Geometry: final body of the model. Coordinates: model frame, mm. A direction names the side the tool comes from. Give positions to 0.01 mm unless a question says otherwise; leave off trailing zeros. Loops run counter-clockwise (first coordinate to the right, second up) from the corner with the lowest first, then second, coordinate; pieces in that order, holes last. Notation, with made-up numbers: (44, 24.5) -> (77, 24.5) arc R24 ccw to (77, 56.5) -> close; hole circle Ø3 at (1, 30). An arc over 180 degrees is marked (long way). Answer in a Markdown table with one row per item. Add a question column.
1) Line query: line 1 (X direction, y = 110, z = 2.9); line 2 (Y direction, x = -268, z = 5.45); line 3 (Y direction, x = -479, z = 2.7). Output: solid intervals per line, ascending. Write a range as from..to.
2) Section query D-D (y = 147). Return the cut outline in (x, z).
3) Section query B-B (x = -372). Return the cut outline in (y, z).
4) First-contact query: P1, Ø2, axis at y = 257, z = 2, coming from the -X side; P2, Ø1.8, axis at y = 100.5, z = 4, coming from the +X side; P3, Ø2, axis at y = 307.5, z = 1, coming from the +X side. Flat tips, straight axial feed; report the tip coordinate or a pass-through.
5) Access query for faces 1 (the flat face through (-345, 205, 6)), 2 (the flat face through (-416.64, 252.094, 2.958)). Directions: +Z, -Z, +X, -X, +Y, -Y. A direction counts if a zero-diameter tool reaches every point of the face in a straight line with its end or side. Return the directions, or none.
6) Draft query along X for faces 3 (the flat face through (-257.967, 389.491, 2.958)), 4 (the flat face through (-199.524, 328.265, 2.958)), 5 (the flat face through (-261.61, 241.79, 2.96)), 6 (the cylindrical face through (-532.244, 297.201, 2.958)). Return one class per face: +X half, -X half, draft (parallel to the pull), parting line (faces both ways), or undercut.
7) Section query A-A (z = 4.65). Return the cut outline in (x, y).
8) Section query C-C (y = 312). Return the cut outline in (x, z), plus the area to 3 significant figures.
```python
from build123d import *

# Parameters (mm, degrees)
BOSS_EXTRUDE1_DEPTH = 6


with BuildPart() as part:
    # Sketch1 → Boss-Extrude1 (new body)
    with BuildSketch(Plane.XY):
        with BuildLine():
            ThreePointArc((-83.576869021, 127.438875406), (-134.094882152, 72.417695218), (-152.4, 0))
            Line((-152.4, 0), (-609.6, 0))
            ThreePointArc((-609.6, 0), (-530.080884891, 301.042215433), (-312.269240574, 523.545682239))
            Line((-312.269240574, 523.545682239), (-83.576869021, 127.438875406))
        make_face()
        with BuildLine():
            ThreePointArc((-154.05140053, 77.394612181), (-149.302779612, 86.2), (-144.05140053, 94.715120257))
            ThreePointArc((-144.05140053, 94.715120257), (-128.363659898, 115.08488527), (-109.821022542, 132.895082707))
            Line((-109.821022542, 132.895082707), (-184.920508076, 262.971207273))
            Line((-184.920508076, 262.971207273), (-310.2, 190.641058886))
            Line((-310.2, 190.641058886), (-320.2, 184.867556195))
            Line((-320.2, 184.867556195), (-320.2, 173.320550811))
            Line((-320.2, 173.320550811), (-320.2, 20))
            Line((-320.2, 20), (-171.235977528, 20))
            ThreePointArc((-171.235977528, 20), (-165.156001883, 49.449520141), (-154.05140053, 77.394612181))
        make_face(mode=Mode.SUBTRACT)
        with BuildLine():
            Line((-340.2, 20), (-589.260689339, 20))
            ThreePointArc((-589.260689339, 20), (-568.194860877, 157.425411141), (-515.535131015, 286.097341284))
            Line((-515.535131015, 286.097341284), (-340.2, 184.867556195))
            Line((-340.2, 184.867556195), (-340.2, 20))
        make_face(mode=Mode.SUBTRACT)
        with BuildLine():
            Line((-330.2, 202.18806427), (-505.535131015, 303.41784936))
            ThreePointArc((-505.535131015, 303.41784936), (-423.458843967, 410.256952977), (-319.272010805, 495.674836073))
            Line((-319.272010805, 495.674836073), (-194.920508076, 280.291715349))
            Line((-194.920508076, 280.291715349), (-330.2, 202.18806427))
        make_face(mode=Mode.SUBTRACT)
    extrude(amount=BOSS_EXTRUDE1_DEPTH)


solid = part.part
```
Evaluation:
| question | item | result |
|---|---|---|
| 1 | line 1 | -599.59..-579.25, -340.2..-320.2, -132.75..-105.48 |
| 1 | line 2 | 0..20, 215.01..238.1, 406.87..446.87 |
| 1 | line 3 | 0..20, 265..288.1, 343.78..377.06 |
| 2 | outline | (-591.61, 0) -> (-570.98, 0) -> (-570.98, 6) -> (-591.61, 6) -> close; (-340.2, 0) -> (-320.2, 0) -> (-320.2, 6) -> (-340.2, 6) -> close; (-117.96, 0) -> (-94.87, 0) -> (-94.87, 6) -> (-117.96, 6) -> close |
| 3 | outline | (0, 0) -> (20, 0) -> (20, 6) -> (0, 6) -> close; (203.23, 0) -> (226.32, 0) -> (226.32, 6) -> (203.23, 6) -> close; (457.43, 0) -> (482.94, 0) -> (482.94, 6) -> (457.43, 6) -> close |
| 4 | P1 | x = -553.24 |
| 4 | P2 | x = -113.77 |
| 4 | P3 | x = -186.96 |
| 5 | face 1 | +Z, +X, -X, +Y, -Y |
| 5 | face 2 | +Z, -Z |
| 6 | face 3 | undercut |
| 6 | face 4 | +X half |
| 6 | face 5 | undercut |
| 6 | face 6 | -X half |
| 7 | outline | (-609.6, 0) -> (-152.4, 0) arc R152.4 cw to (-83.58, 127.44) -> (-312.27, 523.55) arc R609.6 ccw to start; hole (-589.26, 20) -> (-340.2, 20) -> (-340.2, 184.87) -> (-515.54, 286.1) arc R589.6 ccw to start; hole (-505.54, 303.42) -> (-330.2, 202.19) -> (-194.92, 280.29) -> (-319.27, 495.67) arc R589.6 ccw to start; hole (-320.2, 20) -> (-171.24, 20) arc R172.4 cw to (-109.82, 132.9) -> (-184.92, 262.97) -> (-320.2, 184.87) -> close |
| 8 | outline | (-523.71, 0) -> (-500.28, 0) -> (-500.28, 6) -> (-523.71, 6) -> close; (-213.23, 0) -> (-190.13, 0) -> (-190.13, 6) -> (-213.23, 6) -> close |
| 8 | area | 279 mm² |
